Build history of the part. All positions in model axes, mm. A direction names the side the tool comes from. Round coordinates to 2 decimals unless told otherwise and drop trailing zeros. Order: outer loops, then holes, each group sorted by start corner. A loop starts at its lowest first (then second) coordinate and runs counter-clockwise, first axis right, second up. Notation, with made-up numbers: (-16, 35) -> (37, 35) arc R20 ccw to (37, 47) -> close; hole circle Ø2 at (5, -15). An arc over 180 degrees is marked (long way). Answer as a JSON object with one key per item and string values.
Autodesk Inventor part; units mm, degrees
ref_plane "YZ Plane" through (0, 0, 0) normal (1, 0, 0) x (0, 1, 0)
ref_plane "XZ Plane" through (0, 0, 0) normal (0, 1, 0) x (-1, 0, 0)
ref_plane "XY Plane" through (0, 0, 0) normal (0, 0, 1) x (1, 0, 0)
sketch "Sketch2" plane through (0, 0, 0) normal (1, 0, 0) x (0, 1, 0)
  line L0 (0, 0) -> (-3.985, 0)
  line L1 (0, -80.84) -> (0.015, -80.84)
  line L2 (-8.87, -80.84) -> (0, -80.84)
  line L3 (-3.985, -78.84) -> (-8.87, -78.84)
  line L4 (-8.87, -78.84) -> (-8.87, -80.84)
  line L5 (-3.985, -24.34) -> (-3.785, -24.34)
  line L6 (-3.785, -24.34) -> (-3.785, -25.34)
  line L7 (-3.785, -25.34) -> (-3.985, -25.34)
  line L8 (-3.985, -25.34) -> (-3.985, -24.34)
  line L9 (0, 0) -> (0, -80.84)
  line L10 (-6.435, 0) -> (-6.435, -12.64) construction
  line L11 (-6.435, -12.64) -> (0, -12.64) construction
  line L12 (-3.985, 0) -> (-3.985, -24.34)
  line L13 (-3.985, -25.34) -> (-3.985, -78.84)
  line L14 (0, 0) -> (0, -80.84)
  line L15 (-3.985, -1) -> (-3.185, -1)
  line L16 (-3.185, -1) -> (-3.185, -1.9)
  line L17 (-3.185, -1.9) -> (-3.985, -1.9)
  line L18 (-3.985, -1.9) -> (-3.985, -1)
  line L19 (2.8591, -2.1) -> (-4.9211, -2.1) construction
  line L20 (-4.9211, -2.1) -> (-4.9211, -10.99) construction
  line L21 (-4.9211, -10.99) -> (2.8591, -10.99) construction
  line L22 (2.8591, -10.99) -> (2.8591, -2.1) construction
  line L23 (-3.985, -11.19) -> (-3.185, -11.19)
  line L24 (-3.185, -11.19) -> (-3.185, -12.09)
  line L25 (-3.185, -12.09) -> (-3.985, -12.09)
  line L26 (-3.985, -12.09) -> (-3.985, -11.19)
  point P0 (-8.87, -79.84)
  point P1 (-4.9211, -6.545)
  point P2 (-3.585, -1)
  point P3 (-3.985, -12.09)
  dimension "d3" = 1
  dimension "d5" = 0.2
  dimension "d18" = 55.5
  dimension "d21" = 2
  dimension "d22" = 17.74
  dimension "d24" = 12.64
  dimension "d25" = 6.435
  dimension "d26" = 12.7
  dimension "d35" = 0.9
  dimension "d36" = 0.8
  dimension "d38" = 8.89
  dimension "d39" = 0.2
  dimension "d40" = 1
  dimension "d41" = 3.985
  dimension "d45" = 0.2
revolve "Revolution1" add sketch "Sketch2" angle 360 about axis through (0, 0, 0) along (0, 0, -1) contours L9 L2 L4 L3 L13 L7 L6 L5 L12 L25 L24 L23 L17 L16 L15 L0
sketch "Sketch4" plane through (0, 0, -80.84) normal (0, 0, -1) x (-1, 0, 0)
  circle A0 centre (0, 0) radius 6.87 construction
  circle A1 centre (6.87, 0) radius 1.25
  circle A2 centre (0, 0) radius 8.87
  circle A3 centre (-3.435, 5.9496) radius 1.25
  circle A4 centre (-3.435, -5.9496) radius 1.25
  dimension "d28" = 2.5
  dimension "d46" = 2
  dimension "d49" = 360
extrude "Extrusion2" cut sketch "Sketch4" against normal through all contours A1 | A3 | A4
sketch "Sketch5" plane through (0, 0, -80.84) normal (0, 0, -1) x (-1, 0, 0)
  circle A0 centre (6.87, 0) radius 1.25
  circle A1 centre (-3.435, -5.9496) radius 1.25
  circle A2 centre (-3.435, 5.9496) radius 1.25
  circle A3 centre (0, 0) radius 8.87
  circle A4 centre (0, 0) radius 10.87
  dimension "d51" = 2
extrude "Extrusion3" add sketch "Sketch5" along normal blind 2 contours A3 | A4
sketch "Sketch6" plane through (0, 0, 0) normal (0, 0, 1) x (1, 0, 0)
  circle A0 centre (0, 0) radius 3.985
extrude "Extrusion4" add sketch "Sketch6" along normal blind 0.5
chamfer "Chamfer2" distance 0.275 angle 45 1 edges at (-3.985, 0, 0.5)
equation "\"d45\" = d39"
properties part number "FlipperH5055RoundShaft"
1) Probe L1, parallel to Z at x = 5, y = -6.25; L2, parallel to Z at x = -3.75, y = 8.75; L3, parallel to Y at x = -6.87, z = -80.65. List the from-to ranges inside material, lowest first. Write a range as from..to.
Checked values:
{"L1": "z = -82.84..-78.84", "L2": "z = -82.84..-80.84", "L3": "y = -5.61..-1.25, 1.25..5.61"}
2) Cut at A-A, the plane x = -6.87. Give the cut face in (y, z).
Checked values:
{"outline": "(-8.42, -82.84) -> (-1.25, -82.84) -> (-1.25, -78.84) -> (-5.61, -78.84) -> (-5.61, -80.84) -> (-8.42, -80.84) -> close; (1.25, -82.84) -> (8.42, -82.84) -> (8.42, -80.84) -> (5.61, -80.84) -> (5.61, -78.84) -> (1.25, -78.84) -> close"}
3) Cut at B-B, the plane z = -59. Give the cut face in (x, y) (3 decimals).
Checked values:
{"outline": "circle Ø7.97 at (0, 0)"}
4) Pull direction Y, two halves, no side cores. Call faces 4 (the face through (2, 3, -11.19)), 5 (the face through (3.6, 7.19, -80.87)), 6 (the face through (-1.2, -3.8, -6.6)), 7 (the face through (3.6, -7.19, -80.81)): pulls with the +Y half, pulls with the -Y half, needs draft (parallel to the pull), parting line crosses it, or undercut.
Checked values:
{"face 4": "needs draft", "face 5": "undercut", "face 6": "parting line crosses it", "face 7": "undercut"}
5) Cut at C-C, the plane x = 6.5. Give the cut face in (y, z), plus the area to 3 significant figures.
Checked values:
{"outline": "(-8.71, -82.84) -> (8.71, -82.84) -> (8.71, -80.84) -> (6.04, -80.84) -> (6.04, -78.84) -> (-6.04, -78.84) -> (-6.04, -80.84) -> (-8.71, -80.84) -> close", "area": "59.0 mm²"}
6) Flat gauge pins, fed straight in: pin 1 Ø10 at (x, z) = (0.5, -14) entering from +Y (3 decimals); pin 2 Ø1.5 at (y, z) = (2.5, -25.5) entering from -X; pin 3 Ø6 at (y, z) = (1.5, -23) entering from -X (3 decimals). Where does each tip first touch, or does it go through?
Checked values:
{"pin 1": "stops at y = 3.985", "pin 2": "stops at x = -3.58", "pin 3": "stops at x = -3.985"}
7) Which spindle directions (+Z, -Z, +X, -X, +Y, -Y) get a long thin tool onto all of the face, cutting with end or side? Do faces 1 (the face through (-1.2, -3.8, -18.3)), 2 (the face through (-5.62, 0.05, -80.87)), 3 (the face through (-0.957, -3.038, -1.456)). Say none if no direction does.
Checked values:
{"face 1": "+Z", "face 2": "+Z, -Z", "face 3": "none"}
